```python
from build123d import *

# Parameters (mm, degrees)
SKETCH_1_W          = 90
SKETCH_1_H          = 63
EXTRUDE_1_DEPTH     = 3
FILLET_1_R          = 3
SKETCH_2_R          = 1.5
SKETCH_2_R_2        = 2
CUT_EXTRUDE_1_DEPTH = 10
CUT_EXTRUDE_2_DEPTH = 10


with BuildPart() as part:
    # 草图1 → 凸台-拉伸1 (new body)
    with BuildSketch(Plane(origin=(0, 0, 0), x_dir=(1, 0, 0), z_dir=(0, 1, 0))):
        Rectangle(SKETCH_1_W, SKETCH_1_H)
    extrude(amount=EXTRUDE_1_DEPTH)

    # 圆角1
    fillet_1_edges = [part.edges().sort_by_distance(p)[0] for p in [
        (45, 1.5, 31.5),
        (-45, 1.5, 31.5),
        (-45, 1.5, -31.5),
        (45, 1.5, -31.5),
    ]]
    fillet(fillet_1_edges, radius=FILLET_1_R)

    # 草图2 → 切除-拉伸1 (cut)
    with BuildSketch(Plane(origin=(0, 3, 0), x_dir=(1, 0, 0), z_dir=(0, 1, 0))):
        with Locations(Location((-40, 10, 0), (0, 0, 270))):
            Circle(SKETCH_2_R)
        with Locations(Location((-40, -10, 0), (0, 0, 270))):
            Circle(SKETCH_2_R)
        with Locations(Location((40, -10, 0), (0, 0, 270))):
            Circle(SKETCH_2_R)
        with Locations(Location((40, 10, 0), (0, 0, 270))):
            Circle(SKETCH_2_R)
        with Locations(Location((-22, -26.5, 0), (0, 0, 270))):
            Circle(SKETCH_2_R_2)
        with Locations(Location((-14, -26.5, 0), (0, 0, 270))):
            Circle(SKETCH_2_R_2)
        with Locations(Location((14, -26.5, 0), (0, 0, 270))):
            Circle(SKETCH_2_R_2)
        with Locations(Location((22, -26.5, 0), (0, 0, 270))):
            Circle(SKETCH_2_R_2)
        with Locations(Location((22, 26.5, 0), (0, 0, 270))):
            Circle(SKETCH_2_R_2)
        with Locations(Location((14, 26.5, 0), (0, 0, 270))):
            Circle(SKETCH_2_R_2)
        with Locations(Location((-14, 26.5, 0), (0, 0, 270))):
            Circle(SKETCH_2_R_2)
        with Locations(Location((-22, 26.5, 0), (0, 0, 270))):
            Circle(SKETCH_2_R_2)
    extrude(amount=-CUT_EXTRUDE_1_DEPTH, mode=Mode.SUBTRACT)

    # 草图4 → 切除-拉伸2 (cut)
    with BuildSketch(Plane(origin=(0, 3, 0), x_dir=(1, 0, 0), z_dir=(0, 1, 0))):
        with BuildLine():
            Line((16.70561704, -19), (4.5, -19))
            ThreePointArc((4.5, -19), (3.085786438, -18.414213562), (2.5, -17))
            Line((2.5, -17), (2.5, -6.782494944))
            ThreePointArc((2.5, -6.782494944), (3.653707073, -4.970372354), (5.783788282, -5.248908414))
            Line((5.783788282, -5.248908414), (17.989405322, -15.466413469))
            ThreePointArc((17.989405322, -15.466413469), (18.585400679, -17.682944704), (16.70561704, -19))
        make_face()
        with BuildLine():
            Line((14.510594678, -6.033586531), (26.716211718, -16.251091586))
            ThreePointArc((26.716211718, -16.251091586), (28.846292927, -16.529627646), (30, -14.717505056))
            Line((30, -14.717505056), (30, -4.5))
            ThreePointArc((30, -4.5), (29.414213562, -3.085786438), (28, -2.5))
            Line((28, -2.5), (15.79438296, -2.5))
            ThreePointArc((15.79438296, -2.5), (13.914599321, -3.817055296), (14.510594678, -6.033586531))
        make_face()
        with BuildLine():
            Line((28, 2.5), (15.79438296, 2.5))
            ThreePointArc((15.79438296, 2.5), (13.914599321, 3.817055296), (14.510594678, 6.033586531))
            Line((14.510594678, 6.033586531), (26.716211718, 16.251091586))
            ThreePointArc((26.716211718, 16.251091586), (28.846292927, 16.529627646), (30, 14.717505056))
            Line((30, 14.717505056), (30, 4.5))
            ThreePointArc((30, 4.5), (29.414213562, 3.085786438), (28, 2.5))
        make_face()
        with BuildLine():
            Line((5.783788282, 5.248908414), (17.989405322, 15.466413469))
            ThreePointArc((17.989405322, 15.466413469), (18.585400679, 17.682944704), (16.70561704, 19))
            Line((16.70561704, 19), (4.5, 19))
            ThreePointArc((4.5, 19), (3.085786438, 18.414213562), (2.5, 17))
            Line((2.5, 17), (2.5, 6.782494944))
            ThreePointArc((2.5, 6.782494944), (3.653707073, 4.970372354), (5.783788282, 5.248908414))
        make_face()
        with BuildLine():
            Line((-16.70561704, 19), (-4.5, 19))
            ThreePointArc((-4.5, 19), (-3.085786438, 18.414213562), (-2.5, 17))
            Line((-2.5, 17), (-2.5, 6.782494944))
            ThreePointArc((-2.5, 6.782494944), (-3.653707073, 4.970372354), (-5.783788282, 5.248908414))
            Line((-5.783788282, 5.248908414), (-17.989405322, 15.466413469))
            ThreePointArc((-17.989405322, 15.466413469), (-18.585400679, 17.682944704), (-16.70561704, 19))
        make_face()
        with BuildLine():
            Line((-14.510594678, 6.033586531), (-26.716211718, 16.251091586))
            ThreePointArc((-26.716211718, 16.251091586), (-28.846292927, 16.529627646), (-30, 14.717505056))
            Line((-30, 14.717505056), (-30, 4.5))
            ThreePointArc((-30, 4.5), (-29.414213562, 3.085786438), (-28, 2.5))
            Line((-28, 2.5), (-15.79438296, 2.5))
            ThreePointArc((-15.79438296, 2.5), (-13.914599321, 3.817055296), (-14.510594678, 6.033586531))
        make_face()
        with BuildLine():
            Line((-28, -2.5), (-15.79438296, -2.5))
            ThreePointArc((-15.79438296, -2.5), (-13.914599321, -3.817055296), (-14.510594678, -6.033586531))
            Line((-14.510594678, -6.033586531), (-26.716211718, -16.251091586))
            ThreePointArc((-26.716211718, -16.251091586), (-28.846292927, -16.529627646), (-30, -14.717505056))
            Line((-30, -14.717505056), (-30, -4.5))
            ThreePointArc((-30, -4.5), (-29.414213562, -3.085786438), (-28, -2.5))
        make_face()
        with BuildLine():
            Line((-5.783788282, -5.248908414), (-17.989405322, -15.466413469))
            ThreePointArc((-17.989405322, -15.466413469), (-18.585400679, -17.682944704), (-16.70561704, -19))
            Line((-16.70561704, -19), (-4.5, -19))
            ThreePointArc((-4.5, -19), (-3.085786438, -18.414213562), (-2.5, -17))
            Line((-2.5, -17), (-2.5, -6.782494944))
            ThreePointArc((-2.5, -6.782494944), (-3.653707073, -4.970372354), (-5.783788282, -5.248908414))
        make_face()
    extrude(amount=-CUT_EXTRUDE_2_DEPTH, mode=Mode.SUBTRACT)


solid = part.part
```
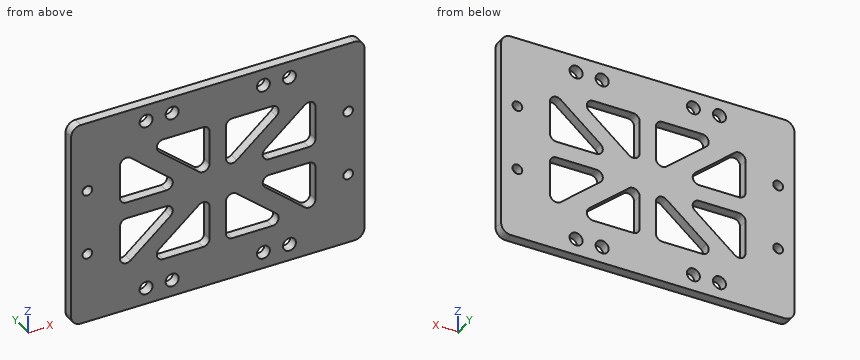
Verification items for the finished model (mm, model axes). Give positions to 0.01 mm unless a question says otherwise; leave off trailing zeros. Loops run counter-clockwise (first coordinate to the right, second up) from the corner with the lowest first, then second, coordinate; pieces in that order, holes last.
1. Section check D-D, the plane y = 0.9. Count the separate pieces of the cut face and the enclosed holes in it, then the cut area to 3 significant figures.
2. Section check C-C, the plane x = -22. Enter the section's corners in (y, z).
3. Section check B-B, the plane x = 40. Enter the section's corners in (y, z).
4. Section check A-A, the plane z = 26.5. Enter the section's corners in (x, y).
5. Thickness scan on line 1 (X direction, y = 1.1, z = 26.5); line 2 (Z direction, x = -21, y = 1.2); line 3 (Z direction, x = -39, y = 0.35). Record the ranges inside material, lowest first.
Geometry says:
1. separate pieces: 1
1. enclosed holes: 20
1. area: 4,320 mm2
2. outline: (0, -31.5) - (3, -31.5) - (3, -28.5) - (0, -28.5) - close; (0, -24.5) - (3, -24.5) - (3, -12.3) - (0, -12.3) - close; (0, -2.5) - (3, -2.5) - (3, 2.5) - (0, 2.5) - close; (0, 12.3) - (3, 12.3) - (3, 24.5) - (0, 24.5) - close; (0, 28.5) - (3, 28.5) - (3, 31.5) - (0, 31.5) - close
3. outline: (0, -31.5) - (3, -31.5) - (3, -11.5) - (0, -11.5) - close; (0, -8.5) - (3, -8.5) - (3, 8.5) - (0, 8.5) - close; (0, 11.5) - (3, 11.5) - (3, 31.5) - (0, 31.5) - close
4. outline: (-45, 0) - (-24, 0) - (-24, 3) - (-45, 3) - close; (-20, 0) - (-16, 0) - (-16, 3) - (-20, 3) - close; (-12, 0) - (12, 0) - (12, 3) - (-12, 3) - close; (16, 0) - (20, 0) - (20, 3) - (16, 3) - close; (24, 0) - (45, 0) - (45, 3) - (24, 3) - close
5. line 1: x = -45 to -24, -20 to -16, -12 to 12, 16 to 20, 24 to 45
5. line 2: z = -31.5 to -28.23, -24.77 to -11.47, -2.5 to 2.5, 11.47 to 24.77, 28.23 to 31.5
5. line 3: z = -31.5 to -11.12, -8.88 to 8.88, 11.12 to 31.5
